```python
from build123d import *

# Parameters (mm, degrees)
CUT_EXTRUDE_1_DEPTH = 1.5
FILLET_1_R          = 0.3
CHAMFER_1_SIZE      = 1


with BuildPart() as part:
    # Эскиз1 → Повернуть1 (revolve)
    with BuildSketch(Plane.XY):
        with BuildLine():
            Line((0, 0), (0, 3.625))
            ThreePointArc((0, 3.625), (0.908821487, 4.451033224), (2.1, 4.75))
            Line((2.1, 4.75), (2.6, 4.75))
            Line((2.6, 4.75), (2.6, 2.5))
            Line((2.6, 2.5), (14.6, 2.5))
            Line((14.6, 2.5), (14.6, 0))
            Line((14.6, 0), (0, 0))
        make_face()
    revolve(axis=Axis((14.6, 0, 0), (-1, 0, 0)))

    # Эскиз2 → Вырез-Вытянуть1 (cut)
    with BuildSketch(Plane.ZY):
        Polygon((0.866025404, 1.5), (-0.866025404, 1.5), (-1.732050808, 0), (-0.866025404, -1.5), (0.866025404, -1.5), (1.732050808, 0), align=None)
    extrude(amount=-CUT_EXTRUDE_1_DEPTH, mode=Mode.SUBTRACT)

    # Скругление1
    fillet_1_edges = [part.edges().sort_by_distance(p)[0] for p in [
        (2.6, -2.5, 0),
        (2.6, -4.75, 0),
    ]]
    fillet(fillet_1_edges, radius=FILLET_1_R)

    # Фаска1
    chamfer_1_edges = [part.edges().sort_by_distance(p)[0] for p in [
        (14.6, -2.5, 0),
    ]]
    chamfer(chamfer_1_edges, length=CHAMFER_1_SIZE)


solid = part.part
```
CAD build for the part. Positions are in the model's coordinates, mm. A direction names the side the tool comes from. Give positions to 0.01 mm unless a question says otherwise; leave off trailing zeros. Loops run counter-clockwise (first coordinate to the right, second up) from the corner with the lowest first, then second, coordinate; pieces in that order, holes last. Notation, with made-up numbers: (-31.75, -32) - (-5.75, -32) arc R14 ccw to (-5.75, -28) - close; hole circle Ø8 at (-29.5, 80). An arc over 180 degrees is marked (long way). Put each result on its own line as item: value.
Q1. Mould opens along Z. For faces 4 (the face through (0.74, 0.74, 1.305)), 5 (the face through (8.32, -0.54, 2.44)), 6 (the face through (1.5, 0, 0)), 7 (the face through (0, -2, 0)) say: pulls with the +Z half, pulls with the -Z half, needs draft (parallel to the pull), parting line crosses it, or undercut.
Filled in:
face 4: undercut
face 5: parting line crosses it
face 6: undercut
face 7: needs draft
Q2. Tool access for faces 1 (the face through (1, 1.5, 0)), 2 (the face through (2.6, 0, 3)), 3 (the face through (14.6, 0, 0)): list every direction of +Z, -Z, +X, -X, +Y, -Y with a clear straight run to the whole face (end or side of a thin tool).
Filled in:
face 1: -X
face 2: +X
face 3: +Z, -Z, +X, +Y, -Y
Q3. Flat gauge pins, fed straight in: pin 1 (0.8 mm diameter, centred on x = 1, z = 0, fed in from -Y); pin 2 (1.5 mm diameter, centred on x = 6.5, y = -2, fed in from -Z); pin 3 (1.5 mm diameter, centred on x = 5, z = -2, fed in from +Y). Where does each tip first touch, or does it go through?
Filled in:
pin 1: stops at y = -4.65
pin 2: stops at z = -2.17
pin 3: stops at y = 2.17
Q4. Slice it at A-A (x = 10). Give the cut face in (y, z).
Filled in:
outline: circle Ø5 at (0, 0)
Q5. Probe line 1 along X through (y, z) = (-0.5, -0.75); line 2 along X through (y, z) = (2.25, 2.25); line 3 along Y through (x, z) = (3.5, 0). List the from-to ranges inside material, lowest first.
Filled in:
line 1: x = 1.5 to 14.6
line 2: x = 0 to 2.6
line 3: y = -2.5 to 2.5
